Source: three-view drawing plus pictorial views. Frame: mm from the lowest corner of the part. Give positions to 0.01 mm unless a question says otherwise; leave off trailing zeros. Write each loop counter-clockwise with the first axis right and the second up, starting at its lowest first coordinate (ties: lowest second). Pieces come first, ordered by that corner, then holes.
Q1. Cut plane A-A on x = 184. Return the cut outline in (y, z).
Q2. Cut plane C-C on y = 90. Return the cut outline in (x, z) (1 decimal), plus the area to 3 significant figures.
Q3. Cut plane B-B on z = 7. Return the cut outline in (x, y) (1 decimal).
Q4. Pin query (flat end, axial travel): pin 1 (1.5 mm diameter, centred on x = 237.5, z = 1, fed in from -Y); pin 2 (5 mm diameter, centred on y = 112, z = 4.5, fed in from -X) (1 decimal); pin 3 (6 mm diameter, centred on y = 143.5, z = 3, fed in from -X); pin 4 (8 mm diameter, centred on x = 246, y = 188, fed in from -Z). Return the tip coordinate at first contact, or that it passes through.
Q5. Cut plane D-D on y = 32. Return the cut outline in (x, z) (1 decimal).
Q6. Line query: L1, parallel to X at y = 97.5, z = 1.25 (1 decimal); L2, parallel to Y at x = 130, z = 5.25 (1 decimal); L3, parallel to Y at x = 124.5, z = 5.75 (1 decimal). Output: solid intervals per line, ascending.
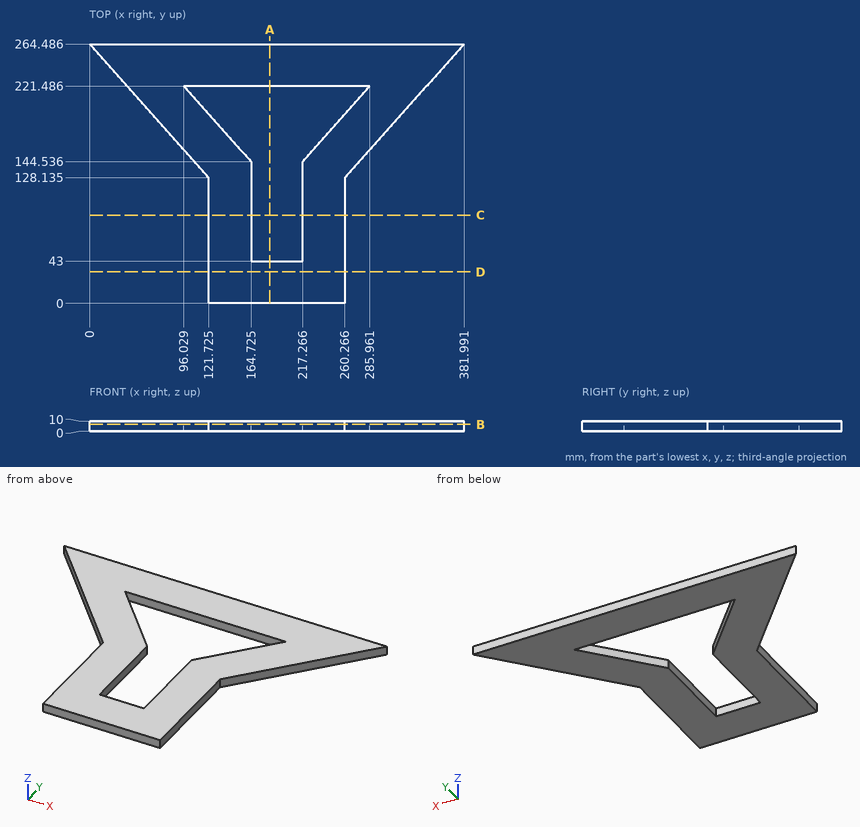
Data:
1. outline: (0, 0) - (43, 0) - (43, 10) - (0, 10) - close; (221.49, 0) - (264.49, 0) - (264.49, 10) - (221.49, 10) - close
2. outline: (121.7, 0) - (164.7, 0) - (164.7, 10) - (121.7, 10) - close; (217.3, 0) - (260.3, 0) - (260.3, 10) - (217.3, 10) - close
2. area: 860 mm2
3. outline: (0, 264.5) - (121.7, 128.1) - (121.7, 0) - (260.3, 0) - (260.3, 128.1) - (382, 264.5) - close; hole (96, 221.5) - (164.7, 144.5) - (164.7, 43) - (217.3, 43) - (217.3, 144.5) - (286, 221.5) - close
4. pin 1: stops at y = 0
4. pin 2: stops at x = 121.7
4. pin 3: stops at x = 105.33
4. pin 4: passes through
5. outline: (121.7, 0) - (260.3, 0) - (260.3, 10) - (121.7, 10) - close
6. L1: x = 121.7 to 164.7, 217.3 to 260.3
6. L2: y = 0 to 183.4, 221.5 to 264.5
6. L3: y = 0 to 189.6, 221.5 to 264.5
